The model under review builds one solid part; all positions refer to its coordinate system, in mm. Face numbers are marked on the shaded views. A direction names the side the tool comes from. Round coordinates to 2 decimals unless told otherwise and drop trailing zeros. Write each loop counter-clockwise with the first axis right and the second up, starting at its lowest first coordinate (ties: lowest second). Pieces come first, ordered by that corner, then holes. Notation, with made-up numbers: (73.25, 0.5) -> (114.25, 0.5) arc R23 cw to (114.25, 33.5) -> close; hole circle Ø1 at (65, 5.5). An arc over 180 degrees is marked (long way). Return JSON: item names as keys, results as strings. Group by question number.
1. Take a section at C-C, the plane x = -7. Write out the cut boundary in (y, z), then the cut area to 3 significant figures.
2. Take a section at D-D, the plane z = 92.5. Write out the cut boundary in (x, y), then the cut area to 3 significant figures.
3. Tool access review of the marked faces 1 and 2: name each direction out of +Z, -Z, +X, -X, +Y, -Y from which nothing blocks a thin tool from reaching the whole face with its end or side.
4. Take a section at A-A, the plane y = 0. Write out the cut boundary in (x, z), then the cut area to 3 significant figures.
5. Clearance check with flat-ended pins moving along their axes: P1, Ø1.9, axis at x = -11, y = 7, coming from the -Z side; P2, Ø12, axis at x = 12.34, y = -6.95, coming from the +Z side; P3, Ø4, axis at y = 11, z = 36, coming from the +X side; P4, Ø12, axis at x = 8.5, z = 24.5, coming from the -Y side. State where each tip first meets the part, or that it passes through.
6. For line 1 along Z through (x, y) = (8, 13); line 2 along Z through (x, y) = (-2, -12); line 3 along X through (y, z) = (6.5, 7), list the stretches that pass through material, from the lowest coordinate up. Write a range as from..to.
7. Take a section at B-B, the plane x = 1.5. Write out the cut boundary in (y, z), then the cut area to 3 significant figures.
from build123d import *

# Parameters (mm, degrees)
F0_R     = 12.7
F1_DEPTH = 127.508
F2_R     = 19.05
F3_DEPTH = 6.35
F4_R     = 3.822156
F5_DEPTH = 7.112


with BuildPart() as f1:
    # F0 (on Top) → F1 (new body)
    with BuildSketch(Plane.XY):
        Circle(F0_R)
    extrude(amount=F1_DEPTH)

    # F2 (on Top) → F3 (join)
    with BuildSketch(Plane.XY):
        Circle(F2_R)
    extrude(amount=F3_DEPTH)

    # F4 (on Top) → F5 (cut)
    with BuildSketch(Plane.XY):
        with Locations((12.194332, 7.214257)):
            Circle(F4_R)
        with Locations((-0.150564, 14.16773)):
            Circle(F4_R)
        with Locations((-12.344896, 6.953473)):
            Circle(F4_R)
        with Locations((-12.194332, -7.214257)):
            Circle(F4_R)
        with Locations((0.150564, -14.16773)):
            Circle(F4_R)
        with Locations((12.344896, -6.953473)):
            Circle(F4_R)
    extrude(amount=F5_DEPTH, mode=Mode.SUBTRACT)


solid = f1.part
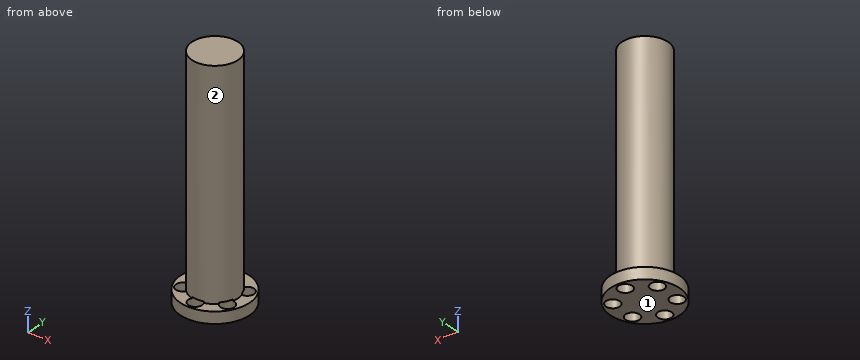
Output:
{
 "1": {"outline": "(-17.72, 0) -> (17.72, 0) -> (17.72, 6.35) -> (10.6, 6.35) -> (10.6, 127.51) -> (-10.6, 127.51) -> (-10.6, 6.35) -> (-17.72, 6.35) -> close", "area": "2,790 mm^2"},
 "2": {"outline": "circle Ø25.4 at (0, 0)", "area": "507 mm^2"},
 "3": {"face 1": "-Z, +X, -X, +Y, -Y", "face 2": "+Z"},
 "4": {"outline": "(-19.05, 0) -> (19.05, 0) -> (19.05, 6.35) -> (12.7, 6.35) -> (12.7, 127.51) -> (-12.7, 127.51) -> (-12.7, 6.35) -> (-19.05, 6.35) -> close", "area": "3,320 mm^2"},
 "5": {"P1": "stops at z = 7.11", "P2": "stops at z = 127.51", "P3": "stops at x = 8.96", "P4": "stops at y = -12.45"},
 "6": {"line 1": "z = 0..6.35", "line 2": "z = 7.11..127.51", "line 3": "x = -8.55..8.44"},
 "7": {"outline": "(-18.99, 0) -> (-17.74, 0) -> (-17.74, 6.35) -> (-18.99, 6.35) -> close; (-12.61, 7.11) -> (-10.59, 7.11) -> (-10.59, 0) -> (10.72, 0) -> (10.72, 7.11) -> (12.61, 7.11) -> (12.61, 127.51) -> (-12.61, 127.51) -> close; (17.62, 0) -> (18.99, 0) -> (18.99, 6.35) -> (17.62, 6.35) -> close", "area": "3,200 mm^2"}
}
